```python
from build123d import *

# Parameters (mm, degrees)
F1_DEPTH    = 25.4
F2_T1_DEPTH = 31.742344746


# Not quite as in the source:
# - a fillet or chamfer that OpenCascade refuses, or shapes differently, is made with other operations: its cross-section is extruded or revolved along the edge and cut away or added


with BuildPart() as f1:
    # F0 (on Front) → F1 (new body)
    with BuildSketch(Plane.XZ):
        with BuildLine():
            Line((1.2633143634, 15.3614934534), (0, 0))
            Line((0, 0), (50.8, 0))
            Line((50.8, 0), (49.5366856366, 15.3614934534))
            ThreePointArc((49.5366856366, 15.3614934534), (25.4, 6.35), (1.2633143634, 15.3614934534))
        make_face()
    extrude(amount=F1_DEPTH)

    # F2: chamfer of 1.27 on 2 edges, made by hand

    # F2_s2 → F2_t1 (cut)
    with BuildSketch(Plane.XZ.offset(-3.171172373)):
        with BuildLine():
            Line((2.2549090841, 14.5889641953), (1.1146425309, 14.1017672287))
            Line((1.1146425309, 14.1017672287), (1.089327991, 14.103849072))
            ThreePointArc((1.089327991, 14.103849072), (1.1860490936, 14.7318712483), (1.2379998236, 15.3635752967))
            Line((1.2379998236, 15.3635752967), (1.2799603535, 15.3806786304))
            ThreePointArc((1.2799603535, 15.3806786304), (1.7575594643, 14.9733769005), (2.2709034327, 14.6086959162))
            Line((2.2709034327, 14.6086959162), (2.2549090841, 14.5889641953))
        make_face()
        with BuildLine():
            Line((48.5450909159, 14.5889641953), (49.6853574691, 14.1017672287))
            Line((49.6853574691, 14.1017672287), (49.710672009, 14.103849072))
            ThreePointArc((49.710672009, 14.103849072), (49.6139509064, 14.7318712483), (49.5620001764, 15.3635752967))
            Line((49.5620001764, 15.3635752967), (49.5200396465, 15.3806786304))
            ThreePointArc((49.5200396465, 15.3806786304), (49.0424405357, 14.9733769005), (48.5290965673, 14.6086959162))
            Line((48.5290965673, 14.6086959162), (48.5450909159, 14.5889641953))
        make_face()
    extrude(amount=F2_T1_DEPTH, mode=Mode.SUBTRACT)


solid = f1.part
```
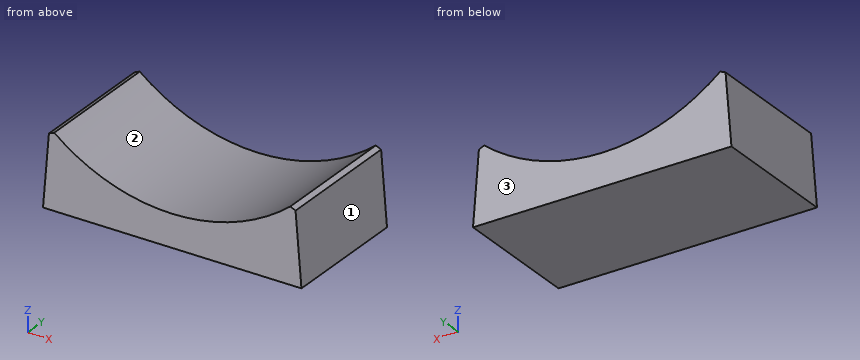
Check sheet for the modelled part. Datum: model origin and axes. Units: mm. Face numbers are marked on the shaded views. Round coordinates to 2 decimals unless told otherwise and drop trailing zeros. Write each loop counter-clockwise with the first axis right and the second up, starting at its lowest first coordinate (ties: lowest second). Pieces come first, ordered by that corner, then holes. Notation, with made-up numbers: (24.5, 67) -> (43.5, 67) arc R25 cw to (43.5, 86) -> close; hole circle Ø2 at (-33, -9.5). An arc over 180 degrees is marked (long way). One line per question, with ' | ' between items. Start each with the question number.
1. Depth check by flat-ended pin: pin 1 (8 mm diameter, centred on y = -12, z = 12, fed in from +X); pin 2 (1 mm diameter, centred on y = -10, z = 7.5, fed in from -X); pin 3 (6 mm diameter, centred on x = 44.5, y = -17, fed in from +Z). Enter the tip coordinate at first touch or a pass-through.
2. Scan lines: line 1 along X through (y, z) = (-17, 13); line 2 along Z through (x, y) = (25, -9.25); line 3 along X through (y, z) = (-23.25, 9.75). Record each from-to range of solid material in increasing order. Write a range as from..to.
3. Sectioned sample at B-B, the plane y = -7.75. Record the cut outline in (x, z).
4. Release check for a two-part mould opening along X. For the marked faces 1, 2 and 3 record: +X half, -X half, draft (parallel to the pull), parting line (faces both ways), or undercut.
5. Sectioned sample at D-D, the plane x = 34.5. Record the cut outline in (y, z), then the cut area to 3 significant figures.
6. Sectioned sample at C-C, the plane z = 7.25. Record the cut outline in (x, y), then the cut area to 3 significant figures.
7. Sectioned sample at A-A, the plane z = 11. Record the cut outline in (x, y).
Taken from the geometry:
1) pin 1: stops at x = 50.14 | pin 2: stops at x = 0.58 | pin 3: stops at z = 13.72
2) line 1: x = 1.07..4.29, 46.51..49.73 | line 2: z = 0..6.35 | line 3: x = 0.8..9.94, 40.86..50
3) outline: (0, 0) -> (50.8, 0) -> (49.64, 14.12) -> (48.59, 14.57) arc R36.83 cw to (2.21, 14.57) -> (1.16, 14.12) -> close
4) face 1: +X half | face 2: undercut | face 3: draft
5) outline: (-25.4, 0) -> (0, 0) -> (0, 7.49) -> (-25.4, 7.49) -> close | area: 190 mm^2
6) outline: (0.6, -25.4) -> (17.31, -25.4) -> (17.31, 0) -> (0.6, 0) -> close; (33.49, -25.4) -> (50.2, -25.4) -> (50.2, 0) -> (33.49, 0) -> close | area: 849 mm^2
7) outline: (0.9, -25.4) -> (7.49, -25.4) -> (7.49, 0) -> (0.9, 0) -> close; (43.31, -25.4) -> (49.9, -25.4) -> (49.9, 0) -> (43.31, 0) -> close
